Can you work these out from the model? Positions are in its coordinate system, mm. Face numbers are marked on the shaded views. Round coordinates to 2 decimals unless told otherwise and drop trailing zeros. Loops run counter-clockwise (first coordinate to the right, second up) from the corner with the lowest first, then second, coordinate; pieces in that order, holes last.
(1) If I drill on line 1 along X through (y, z) = (3.25, 11.5); line 2 along X through (y, z) = (7.5, 24.5); line 3 along Y through (x, z) = (0, 20), over which ranges is the centre line in solid material (lowest first)?
(2) Thinking about a two-plate mould opening in Y: for the marked faces 1, 2, 3 and 4, which applies, released by +Y, released by -Y, zero draft, split by the parting line, or undercut?
(3) I want a section at A-A on x = 0. Write out the boundary of the cut face in (y, z).
(4) Will these pins go through, and if not, where does the flat tip stop? pin 1 Ø1.8 at (x, z) = (-0.5, 13.5) entering from -Y; pin 2 Ø2.5 at (x, z) = (0.5, 17) entering from +Y; pin 3 Ø0.6 at (x, z) = (9, 14) entering from -Y.
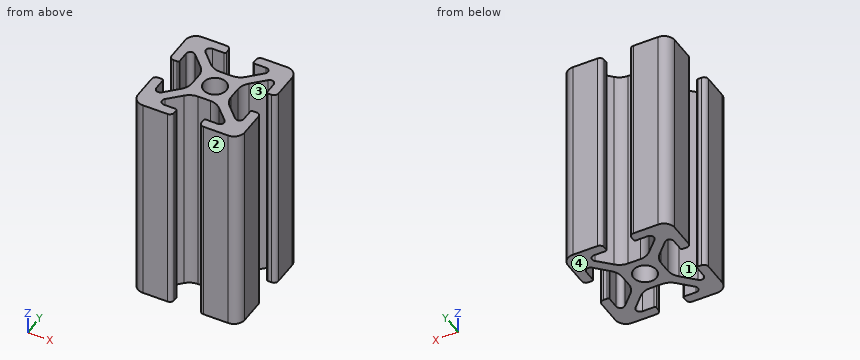
from build123d import *

# Parameters (mm, degrees)
CROQUIS1_R              = 2.15
SALIENTE_EXTRUIR1_DEPTH = 40


with BuildPart() as part:
    # Croquis1 → Saliente-Extruir1 (new body)
    with BuildSketch(Plane.XY):
        with BuildLine():
            Line((3.65, 1.134567107), (3.65, -1.134567107))
            ThreePointArc((3.65, -1.134567107), (3.878361402, -2.282617404), (4.528679656, -3.25588745))
            Line((4.528679656, -3.25588745), (6.868456711, -5.595664505))
            ThreePointArc((6.868456711, -5.595664505), (7.718493077, -5.764747251), (8.2, -5.044121215))
            Line((8.2, -5.044121215), (8.2, -2.87))
            ThreePointArc((8.2, -2.87), (8.287867966, -2.657867966), (8.5, -2.57))
            Line((8.5, -2.57), (9.2, -2.57))
            ThreePointArc((9.2, -2.57), (9.765685425, -2.804314575), (10, -3.37))
            Line((10, -3.37), (10, -8))
            ThreePointArc((10, -8), (9.414213562, -9.414213562), (8, -10))
            Line((8, -10), (3.37, -10))
            ThreePointArc((3.37, -10), (2.804314575, -9.765685425), (2.57, -9.2))
            Line((2.57, -9.2), (2.57, -8.5))
            ThreePointArc((2.57, -8.5), (2.657867966, -8.287867966), (2.87, -8.2))
            Line((2.87, -8.2), (5.044121215, -8.2))
            ThreePointArc((5.044121215, -8.2), (5.764747251, -7.718493077), (5.595664505, -6.868456711))
            Line((5.595664505, -6.868456711), (3.25588745, -4.528679656))
            ThreePointArc((3.25588745, -4.528679656), (2.282617404, -3.878361402), (1.134567107, -3.65))
            Line((1.134567107, -3.65), (-1.134567107, -3.65))
            ThreePointArc((-1.134567107, -3.65), (-2.282617404, -3.878361402), (-3.25588745, -4.528679656))
            Line((-3.25588745, -4.528679656), (-5.595664505, -6.868456711))
            ThreePointArc((-5.595664505, -6.868456711), (-5.764747251, -7.718493077), (-5.044121215, -8.2))
            Line((-5.044121215, -8.2), (-2.87, -8.2))
            ThreePointArc((-2.87, -8.2), (-2.657867966, -8.287867966), (-2.57, -8.5))
            Line((-2.57, -8.5), (-2.57, -9.2))
            ThreePointArc((-2.57, -9.2), (-2.804314575, -9.765685425), (-3.37, -10))
            Line((-3.37, -10), (-8, -10))
            ThreePointArc((-8, -10), (-9.414213562, -9.414213562), (-10, -8))
            Line((-10, -8), (-10, -3.37))
            ThreePointArc((-10, -3.37), (-9.765685425, -2.804314575), (-9.2, -2.57))
            Line((-9.2, -2.57), (-8.5, -2.57))
            ThreePointArc((-8.5, -2.57), (-8.287867966, -2.657867966), (-8.2, -2.87))
            Line((-8.2, -2.87), (-8.2, -5.044121215))
            ThreePointArc((-8.2, -5.044121215), (-7.718493077, -5.764747251), (-6.868456711, -5.595664505))
            Line((-6.868456711, -5.595664505), (-4.528679656, -3.25588745))
            ThreePointArc((-4.528679656, -3.25588745), (-3.878361402, -2.282617404), (-3.65, -1.134567107))
            Line((-3.65, -1.134567107), (-3.65, 1.134567107))
            ThreePointArc((-3.65, 1.134567107), (-3.878361402, 2.282617404), (-4.528679656, 3.25588745))
            Line((-4.528679656, 3.25588745), (-6.868456711, 5.595664505))
            ThreePointArc((-6.868456711, 5.595664505), (-7.718493077, 5.764747251), (-8.2, 5.044121215))
            Line((-8.2, 5.044121215), (-8.2, 2.87))
            ThreePointArc((-8.2, 2.87), (-8.287867966, 2.657867966), (-8.5, 2.57))
            Line((-8.5, 2.57), (-9.2, 2.57))
            ThreePointArc((-9.2, 2.57), (-9.765685425, 2.804314575), (-10, 3.37))
            Line((-10, 3.37), (-10, 8))
            ThreePointArc((-10, 8), (-9.414213562, 9.414213562), (-8, 10))
            Line((-8, 10), (-3.37, 10))
            ThreePointArc((-3.37, 10), (-2.804314575, 9.765685425), (-2.57, 9.2))
            Line((-2.57, 9.2), (-2.57, 8.5))
            ThreePointArc((-2.57, 8.5), (-2.657867966, 8.287867966), (-2.87, 8.2))
            Line((-2.87, 8.2), (-5.044121215, 8.2))
            ThreePointArc((-5.044121215, 8.2), (-5.764747251, 7.718493077), (-5.595664505, 6.868456711))
            Line((-5.595664505, 6.868456711), (-3.25588745, 4.528679656))
            ThreePointArc((-3.25588745, 4.528679656), (-2.282617404, 3.878361402), (-1.134567107, 3.65))
            Line((-1.134567107, 3.65), (1.134567107, 3.65))
            ThreePointArc((1.134567107, 3.65), (2.282617404, 3.878361402), (3.25588745, 4.528679656))
            Line((3.25588745, 4.528679656), (5.595664505, 6.868456711))
            ThreePointArc((5.595664505, 6.868456711), (5.764747251, 7.718493077), (5.044121215, 8.2))
            Line((5.044121215, 8.2), (2.87, 8.2))
            ThreePointArc((2.87, 8.2), (2.657867966, 8.287867966), (2.57, 8.5))
            Line((2.57, 8.5), (2.57, 9.2))
            ThreePointArc((2.57, 9.2), (2.804314575, 9.765685425), (3.37, 10))
            Line((3.37, 10), (8, 10))
            ThreePointArc((8, 10), (9.414213562, 9.414213562), (10, 8))
            Line((10, 8), (10, 3.37))
            ThreePointArc((10, 3.37), (9.765685425, 2.804314575), (9.2, 2.57))
            Line((9.2, 2.57), (8.5, 2.57))
            ThreePointArc((8.5, 2.57), (8.287867966, 2.657867966), (8.2, 2.87))
            Line((8.2, 2.87), (8.2, 5.044121215))
            ThreePointArc((8.2, 5.044121215), (7.718493077, 5.764747251), (6.868456711, 5.595664505))
            Line((6.868456711, 5.595664505), (4.528679656, 3.25588745))
            ThreePointArc((4.528679656, 3.25588745), (3.878361402, 2.282617404), (3.65, 1.134567107))
        make_face()
        Circle(CROQUIS1_R, mode=Mode.SUBTRACT)
    extrude(amount=SALIENTE_EXTRUIR1_DEPTH)


solid = part.part
Filled sheet:
1. line 1: x = -9.99 to -8.2, -4.52 to 4.52, 8.2 to 9.99
1. line 2: x = -10 to -5.82, 5.82 to 10
1. line 3: y = -3.65 to -2.15, 2.15 to 3.65
2. face 1: undercut
2. face 2: released by -Y
2. face 3: undercut
2. face 4: zero draft
3. outline: (-3.65, 0) - (-2.15, 0) - (-2.15, 40) - (-3.65, 40) - close; (2.15, 0) - (3.65, 0) - (3.65, 40) - (2.15, 40) - close
4. pin 1: stops at y = -3.66
4. pin 2: stops at y = 3.71
4. pin 3: stops at y = -9.87
